Part model, mm, in its own coordinate system. A direction names the side the tool comes from. Give positions to 0.01 mm unless a question says otherwise; leave off trailing zeros. Write each loop counter-clockwise with the first axis right and the second up, starting at its lowest first coordinate (ties: lowest second). Pieces come first, ordered by that corner, then holes. Notation, with made-up numbers: (52.25, 3.5) - (83.25, 3.5) arc R34 ccw to (83.25, 38.5) - close; hole circle Ø9 at (13, -14). An arc over 180 degrees is marked (long way). Answer as a JSON object with one key per item and string values. Group by question number.
Autodesk Inventor part; units mm, degrees
ref_plane "YZ Plane" through (0, 0, 0) normal (1, 0, 0) x (0, 1, 0)
ref_plane "XZ Plane" through (0, 0, 0) normal (0, 1, 0) x (-1, 0, 0)
ref_plane "XY Plane" through (0, 0, 0) normal (0, 0, 1) x (1, 0, 0)
sketch "Sketch1" plane through (0, 0, 0) normal (0, 0, 1) x (1, 0, 0)
  line L0 (0, 0) -> (31.75, 0)
  line L1 (31.75, 0) -> (31.75, 50.8)
  line L2 (0, 50.8) -> (0, 0)
  line L3 (28.575, 50.8) -> (28.575, 3.175)
  line L4 (28.575, 3.175) -> (3.175, 3.175)
  line L5 (3.175, 3.175) -> (3.175, 50.8)
  line L6 (0, 50.8) -> (3.175, 50.8)
  line L7 (28.575, 50.8) -> (31.75, 50.8)
  dimension "d0" = 50.8
  dimension "d1" = 31.75
  dimension "d2" = 3.175
  dimension "d3" = 3.175
  dimension "d4" = 3.175
extrude "Extrusion1" add sketch "Sketch1" along normal blind 50.8
sketch "Sketch2" plane through (31.75, 0, 0) normal (1, 0, 0) x (0, 0, -1)
  line L0 (-50.8, 50.8) -> (-50.8, 0)
  line L1 (0, 0) -> (0, 50.8)
  line L2 (0, 50.8) -> (-50.8, 50.8)
  line L3 (0, 3.175) -> (-50.8, 3.175)
  circle A0 centre (-25.4, 31.75) radius 14.2875
  arc A1 (-6.749, 35.6286) -> (-44.051, 35.6286) centre (-25.4, 31.75) ccw
  line L4 (-44.051, 35.6286) -> (-50.8, 3.175)
  line L5 (-6.749, 35.6286) -> (0, 3.175)
  dimension "d7" = 28.575
  dimension "d8" = 25.4
  dimension "d9" = 19.05
extrude "Extrusion2" cut sketch "Sketch2" against normal blind 50.8 contours L2 A1 L4 L0 | L2 L1 L5 A1 | A0
sketch "Sketch3" plane through (3.175, 3.175, 50.8) normal (0, 1, 0) x (1, 0, 0)
  line L0 (0, 0) -> (25.4, 0)
  line L1 (25.4, 50.8) -> (25.4, 0)
  line L2 (25.4, 50.8) -> (0, 50.8)
  circle A0 centre (12.7, 38.1) radius 3.175
  circle A1 centre (12.7, 12.7) radius 3.175
  line L3 (0, 50.8) -> (0, 0)
  point P0 (-3.175, 50.8)
  dimension "d12" = 6.35
  dimension "d13" = 6.35
  dimension "d14" = 12.7
  dimension "d15" = 12.7
  dimension "d16" = 12.7
  dimension "d17" = 12.7
  dimension "d20" = 25.4
extrude "Extrusion3" cut sketch "Sketch3" against normal blind 50.8 contours A0 | A1
equation "\"d3\" = d2"
equation "\"d4\" = d2"
equation "\"d12\" = d13"
equation "\"d15\" = 0.5 * d20"
equation "\"d16\" = d14"
equation "\"d17\" = d15"
properties part number "apendage bearing braket"
1) Two-plate mould, pull along X, no slides. Class faces 1 (the cylindrical face through (17.58, 1.61, 35.42)), 2 (the cylindrical face through (1.61, 17.802, 28.497)), 3 (the flat face through (0, 14, 25)), 4 (the flat face through (28.575, 17, 25)): +X half, -X half, draft (parallel to the pull), parting line (faces both ways), or undercut.
2) Drop flat-ended pins along their axis: P1, Ø24, axis at y = 26.5, z = 19, coming from the +X side; P2, Ø5, axis at x = 26, z = 12.5, coming from the +Y side (3 decimals). Give the stop position or say it passes through.
3) Which spindle directions (+Z, -Z, +X, -X, +Y, -Y) get a long thin tool onto all of the face, cutting with end or side? Do faces 5 (the flat face through (16, 2, 0)), 6 (the flat face through (3.175, 16, 25)). Say none if no direction does.
4) Saw through at D-D (x = 14). List the corners of the cut face in (y, z) (3 decimals).
5) Drill centre lines: line 1 along Y through (x, z) = (30, 25); line 2 along X through (y, z) = (48, 26.5) (3 decimals); line 3 along X through (y, z) = (1.05, 12.7). Where is each one in solid material? Low to high. Write a range as from..to.
6) Saw through at B-B (z = 25.4). State how many separate pieces and enclosed holes the cut face has, and give its area (3 significant figures).
Checks:
{
 "1": {"face 1": "undercut", "face 2": "draft", "face 3": "-X half", "face 4": "undercut"},
 "2": {"P1": "x = 31.75", "P2": "y = 3.175"},
 "3": {"face 5": "-Z, +X, -X, +Y, -Y", "face 6": "+Z, -Z, +Y"},
 "4": {"outline": "(0, 0) - (3.175, 0) - (3.175, 10.138) - (0, 10.138) - close; (0, 15.262) - (3.175, 15.262) - (3.175, 35.538) - (0, 35.538) - close; (0, 40.662) - (3.175, 40.662) - (3.175, 50.8) - (0, 50.8) - close"},
 "5": {"line 1": "0..17.47, 46.03..50.8", "line 2": "0..3.175, 28.575..31.75", "line 3": "0..12.7, 19.05..31.75"},
 "6": {"separate pieces": "3", "enclosed holes": "0", "area": "222 mm2"}
}
